Work out the finished part from the listing and answer in its coordinate system (mm). Round coordinates to 2 decimals unless told otherwise and drop trailing zeros. Loops run counter-clockwise (first coordinate to the right, second up) from the corner with the lowest first, then second, coordinate; pieces in that order, holes last. Notation, with made-up numbers: (10.5, -21) - (56.5, -21) arc R36 ccw to (56.5, 16) - close; hole circle Ø4 at (29, 81). An arc over 180 degrees is marked (long way). Answer as CSV lines item,"result". Start each with the question number.
Q1. Section A-A on y = 45.59 is taken. Write down the section's boundary in (x, z).
Q2. Each of these flat-tipped pins is pushed along its axis until it touches: pin 1 Ø2.5 at (x, y) = (198.75, 45.59) entering from +Z; pin 2 Ø1.5 at (x, z) = (6.5, 1) entering from -Y; pin 3 Ø0.9 at (x, z) = (197.5, 1.5) entering from +Y. Where does it stop, or does it pass through?
Q3. Straight lines are drawn through the part: L1, parallel to Y at x = 198.75, z = 0.9; L2, parallel to Y at x = 191, z = 2.8; L3, parallel to X at y = 5, z = 0.5. For each, find the intervals that lie inside material, in ascending order. Write a range as [from, to].
```python
from build123d import *

# Parameters (mm, degrees)
BOSS_EXTRUDE1_DEPTH   = 3
F_4_0MM_DOWEL_HOLE1_D = 4


with BuildPart() as part:
    # Sketch1 → Boss-Extrude1 (new body)
    with BuildSketch(Plane.XY):
        with BuildLine():
            Line((0, 7.34), (0, 83.84))
            ThreePointArc((0, 83.84), (0.878679656, 85.961320344), (3, 86.84))
            Line((3, 86.84), (8, 86.84))
            Line((8, 86.84), (18, 91.18))
            Line((18, 91.18), (184.5, 91.18))
            Line((184.5, 91.18), (194.5, 86.84))
            Line((194.5, 86.84), (199.5, 86.84))
            ThreePointArc((199.5, 86.84), (201.621320344, 85.961320344), (202.5, 83.84))
            Line((202.5, 83.84), (202.5, 7.34))
            ThreePointArc((202.5, 7.34), (201.621320344, 5.218679656), (199.5, 4.34))
            Line((199.5, 4.34), (194.5, 4.34))
            Line((194.5, 4.34), (184.5, 0))
            Line((184.5, 0), (18, 0))
            Line((18, 0), (8, 4.34))
            Line((8, 4.34), (3, 4.34))
            ThreePointArc((3, 4.34), (0.878679656, 5.218679656), (0, 7.34))
        make_face()
    extrude(amount=BOSS_EXTRUDE1_DEPTH)

    # Ø4.0mm Dowel Hole1 (through all)
    with Locations(Plane.XY.offset(3)):
        with Locations((3.75, 45.59), (198.75, 45.59)):
            Hole(F_4_0MM_DOWEL_HOLE1_D / 2)


solid = part.part
```
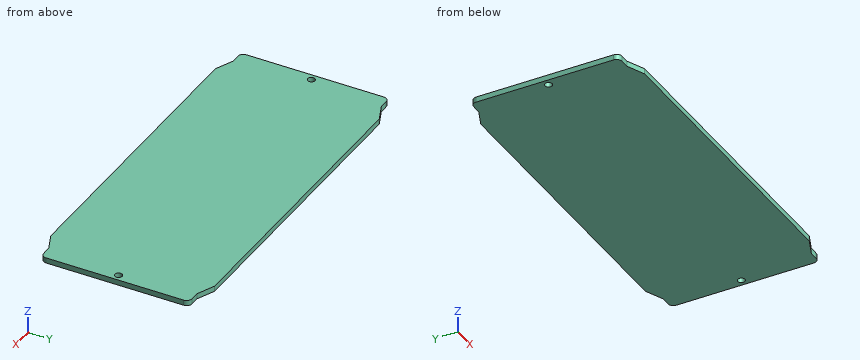
Findings:
1,outline,"(0, 0) - (1.75, 0) - (1.75, 3) - (0, 3) - close; (5.75, 0) - (196.75, 0) - (196.75, 3) - (5.75, 3) - close; (200.75, 0) - (202.5, 0) - (202.5, 3) - (200.75, 3) - close"
2,pin 1,"passes through"
2,pin 2,"stops at y = 4.34"
2,pin 3,"stops at y = 86.84"
3,L1,"y = [4.34, 43.59], [47.59, 86.84]"
3,L2,"y = [2.82, 88.36]"
3,L3,"x = [1.12, 201.38]"
